Build history of the part. All positions in model axes, mm. A direction names the side the tool comes from. Give positions to 0.01 mm unless a question says otherwise; leave off trailing zeros. Order: outer loops, then holes, each group sorted by start corner. A loop starts at its lowest first (then second) coordinate and runs counter-clockwise, first axis right, second up. Notation, with made-up numbers: M -38,25.5 L -17,25.5 A17 cw -17,35.5 Z; hole C 85,23 d5. An arc over 180 degrees is marked long. Use CSV: the item, a comma, the result in double quotes. Start each with the question number.
Item 1: Band-saw the part on A-A on z = 1.75. Write the cut outline in (x, y).
Item 2: Band-saw the part on C-C on y = 13.5. Write the cut outline in (x, z).
Item 3: Band-saw the part on B-B on x = -16. Write the cut outline in (y, z).
Item 4: Band-saw the part on D-D on z = 19.5. Write the cut outline in (x, y).
Item 5: Wall check: line 1 along Z through (x, y) = (-5, 14.75); line 2 along Y through (x, z) = (-11.5, 23.25); line 3 along X through (y, z) = (6.5, 5.25). Give the ranges that are in metal, low to high.
Item 6: Which spindle directions (+Z, -Z, +X, -X, +Y, -Y) get a long thin tool onto all of the face, cutting with end or side? Do faces 1 (the flat face through (-13, 4, 4)), 2 (the flat face through (-4.623, 15.655, 1.972)). Say none if no direction does.
Item 7: Pin check, flat tips, straight feed: P1, Ø3, axis at x = -15.5, z = 12, coming from the +Y side; P2, Ø5, axis at y = 10.5, z = 8, coming from the +X side; P3, Ø8, axis at x = -9.5, z = 17, coming from the +Y side; P4, Ø1, axis at x = -13.5, y = 3, coming from the +Z side. Stop position of each tip, or through.
from build123d import *

# Parameters (mm, degrees)
BOSS_EXTRUDE2_DEPTH = 4
SKETCH4_R           = 4
BOSS_EXTRUDE3_DEPTH = 20
FILLET1_R           = 2
FILLET3_R           = 1


with BuildPart() as part:
    # Sketch1 → Boss-Extrude2 (new body)
    with BuildSketch(Plane.XY):
        Polygon((-0.353108988, 3.18967376), (-0.353108988, 13.18967376), (-9.013363026, 18.18967376), (-17.673617064, 13.18967376), (-17.673617064, 3.18967376), (-9.013363026, -1.81032624), align=None)
    extrude(amount=BOSS_EXTRUDE2_DEPTH)

    # Sketch4 → Boss-Extrude3 (add)
    with BuildSketch(Plane.XY.offset(4)):
        with Locations((-9.013363026, 8.18967376)):
            Circle(SKETCH4_R)
    extrude(amount=BOSS_EXTRUDE3_DEPTH)

    # Fillet1
    fillet1_edges = [part.edges().sort_by_distance(p)[0] for p in [
        (-13.013363026, 8.18967376, 24),
    ]]
    fillet(fillet1_edges, radius=FILLET1_R)

    # Fillet3
    fillet3_edges = [part.edges().sort_by_distance(p)[0] for p in [
        (-13.013363026, 8.18967376, 4),
    ]]
    fillet(fillet3_edges, radius=FILLET3_R)


solid = part.part
Model answer:
1,outline,"M -17.67,3.19 L -9.01,-1.81 L -0.35,3.19 L -0.35,13.19 L -9.01,18.19 L -17.67,13.19 Z"
2,outline,"M -17.14,0 L -0.89,0 L -0.89,4 L -17.14,4 Z"
3,outline,"M 2.22,0 L 14.16,0 L 14.16,4 L 2.22,4 Z"
4,outline,"C -9.01,8.19 d8"
5,line 1,"z = 0 to 4"
5,line 2,"y = 5.64 to 10.74"
5,line 3,"x = -12.64 to -5.39"
6,face 1,"+Z"
6,face 2,"+Z, -Z, +X, +Y"
7,P1,"passes through"
7,P2,"stops at x = -5.01"
7,P3,"stops at y = 12.19"
7,P4,"stops at z = 4"
